```python
from build123d import *

# Parameters (mm, degrees)
F1_W        = 125.7533915341
F1_H        = 114.8591116071
F2_DEPTH    = 20
F3_T        = -5
F5_W        = 42.7649468184
F5_H        = 54.3430875987
F6_DEPTH    = 40
F7_T1_DEPTH = 149.8591116071
F7_T3_DEPTH = 160.7533915341


# Not quite as in the source:
# - a fillet or chamfer that OpenCascade refuses, or shapes differently, is made with other operations: its cross-section is extruded or revolved along the edge and cut away or added


with BuildPart() as f2:
    # F1 (on face) → F2 (new body)
    with BuildSketch(Plane.XY):
        with Locations((-2.1778326482, 3.7721171975)):
            Rectangle(F1_W, F1_H)
    extrude(amount=F2_DEPTH)

    # F3
    f3_openings = [f2.faces().sort_by_distance(p)[0] for p in [
        (-2.177833, 3.772117, 0),
    ]]
    offset(amount=F3_T, openings=f3_openings)

    # F5 (on Top) → F6 (join)
    with BuildSketch(Plane.XY):
        with Locations((1.4939792454, 2.4008983746)):
            Rectangle(F5_W, F5_H)
    extrude(amount=F6_DEPTH)

    # F7: fillet of radius 7 on 4 edges, made by hand

    # F7_s2 → F7_t1 (cut)
    with BuildSketch(Plane.XZ.offset(-78.7016730011)):
        with BuildLine():
            add(Edge.make_bspline(
                [(-58.0545284152, 20), (-65.0545284152, 20), (-65.0545284152, 13)],
                knots=[0, 0, 0, 1, 1, 1], degree=2, weights=[1, 1, 1]))
            Line((-65.0545284152, 13), (-65.0545284152, 20))
            Line((-65.0545284152, 20), (-58.0545284152, 20))
        make_face()
        with BuildLine():
            add(Edge.make_bspline(
                [(60.6988631189, 13), (60.6988631189, 20), (53.6988631189, 20)],
                knots=[0, 0, 0, 1, 1, 1], degree=2, weights=[1, 1, 1]))
            Line((53.6988631189, 20), (60.6988631189, 20))
            Line((60.6988631189, 20), (60.6988631189, 13))
        make_face()
    extrude(amount=F7_T1_DEPTH, mode=Mode.SUBTRACT)

    # F7_s4 → F7_t3 (cut)
    with BuildSketch(Plane.YZ.offset(-82.5545284152)):
        with BuildLine():
            add(Edge.make_bspline(
                [(-53.657438606, 13), (-53.657438606, 20), (-46.657438606, 20)],
                knots=[0, 0, 0, 1, 1, 1], degree=2, weights=[1, 1, 1]))
            Line((-46.657438606, 20), (-53.657438606, 20))
            Line((-53.657438606, 20), (-53.657438606, 13))
        make_face()
        with BuildLine():
            add(Edge.make_bspline(
                [(61.2016730011, 13), (61.2016730011, 20), (54.2016730011, 20)],
                knots=[0, 0, 0, 1, 1, 1], degree=2, weights=[1, 1, 1]))
            Line((54.2016730011, 20), (61.2016730011, 20))
            Line((61.2016730011, 20), (61.2016730011, 13))
        make_face()
    extrude(amount=F7_T3_DEPTH, mode=Mode.SUBTRACT)


solid = f2.part
```
Build history of the part. All positions in model axes, mm. A direction names the side the tool comes from. Round coordinates to 2 decimals unless told otherwise and drop trailing zeros. Loops run counter-clockwise (first coordinate to the right, second up) from the corner with the lowest first, then second, coordinate; pieces in that order, holes last.
Item 1: Which spindle directions (+Z, -Z, +X, -X, +Y, -Y) get a long thin tool onto all of the face, cutting with end or side? Do faces 1 (the face through (1, 29.572, 30)), 2 (the face through (-3, 56.202, 7)), 3 (the face through (22.876, 2, 30)), 4 (the face through (1, -24.771, 30)), 5 (the face through (-19.888, 2, 30)). Say none if no direction does.
Item 2: Pin check, flat tips, straight feed: P1, Ø10, axis at x = -29, z = 17, coming from the -Y side; P2, Ø3, axis at x = 41.5, y = -1.5, coming from the -Z side; P3, Ø22, axis at x = 9.5, z = 33, coming from the -Y side; P4, Ø12, axis at x = 32.5, y = 3, coming from the +Z side. Stop position of each tip, or through.
Item 3: Saw through at A-A (z = 4.5). List the corners of the cut face in (x, y), then the cut area to 3 significant figures.
Item 4: Saw through at B-B (z = 38.5). List the corners of the cut face in (x, y), then the cut area to 3 significant figures.
Item 5: Two-plate mould, pull along Y, no slides. Class faces 6 (the face through (22.876, 2, 7)), 7 (the face through (-3, -53.657, 6)), 8 (the face through (1, 3, 0)), 9 (the face through (1, -24.771, 7)): released by +Y, released by -Y, zero draft, split by the parting line, or undercut.
Item 6: Drill centre lines: line 1 along Y through (x, z) = (-17.5, 11); line 2 along X through (y, z) = (41, 6); line 3 along Y through (x, z) = (44.5, 5.5). Where is each one in solid material? Low to high.
Worked answers:
1. face 1: +Z, +X, -X, +Y
1. face 2: -Z
1. face 3: +Z, +X, +Y, -Y
1. face 4: +Z, +X, -X, -Y
1. face 5: +Z, -X, +Y, -Y
2. P1: stops at y = -53.66
2. P2: stops at z = 15
2. P3: stops at y = -24.77
2. P4: stops at z = 20
3. outline: (-65.05, -53.66) - (60.7, -53.66) - (60.7, 61.2) - (-65.05, 61.2) - close; (-19.89, -24.77) - (22.88, -24.77) - (22.88, 29.57) - (-19.89, 29.57) - close; hole (-60.05, -48.66) - (55.7, -48.66) - (55.7, 56.2) - (-60.05, 56.2) - close
3. area: 4,630 mm2
4. outline: (-19.89, -24.77) - (22.88, -24.77) - (22.88, 29.57) - (-19.89, 29.57) - close
4. area: 2,320 mm2
5. face 6: undercut
5. face 7: released by -Y
5. face 8: zero draft
5. face 9: undercut
6. line 1: y = -53.66 to -48.66, -24.77 to 29.57, 56.2 to 61.2
6. line 2: x = -65.05 to -60.05, 55.7 to 60.7
6. line 3: y = -53.66 to -48.66, 56.2 to 61.2
